```python
from build123d import *

# Parameters (mm, degrees)
F0_W     = 25.4
F0_H     = 28.575
F1_DEPTH = 63.5


with BuildPart() as f1:
    # F0 (on Front) → F1 (new body, symmetric)
    with BuildSketch(Plane.XZ):
        with BuildLine():
            add(Edge.make_bspline(
                [(-41.275, 9.525), (-41.089289, 37.270412), (16.726991, 64.451575), (53.630861, 61.9252)],
                knots=[0, 0, 0, 0, 108.410809, 108.410809, 108.410809, 108.410809], degree=3))
            Line((-41.275, 9.525), (22.225, 9.525))
            Line((22.225, 9.525), (22.225, 30.519339))
            ThreePointArc((22.225, 30.519339), (31.423564, 52.726636), (53.630861, 61.9252))
        make_face()
        Polygon((22.225, 9.525), (-41.275, 9.525), (-41.275, -9.525), (41.275, -9.525), (41.275, 9.525), align=None)
        with BuildLine():
            Line((22.225, 30.519339), (22.225, 9.525))
            Line((22.225, 9.525), (41.275, 9.525))
            Line((41.275, 9.525), (41.275, 30.519339))
            ThreePointArc((41.275, 30.519339), (44.893948, 39.256252), (53.630861, 42.8752))
            Line((53.630861, 42.8752), (60.325, 42.8752))
            Line((60.325, 42.8752), (60.325, 61.9252))
            Line((60.325, 61.9252), (53.630861, 61.9252))
            ThreePointArc((53.630861, 61.9252), (31.423564, 52.726636), (22.225, 30.519339))
        make_face()
        Polygon((60.325, 66.675), (60.325, 61.9252), (60.325, 42.8752), (60.325, 38.1), (85.725, 38.1), (85.725, 66.675), align=None)
        with Locations((98.425, 52.3875)):
            Rectangle(F0_W, F0_H)
    extrude(amount=F1_DEPTH, both=True)


solid = f1.part
```
Work out the finished part from the listing and answer in its coordinate system (mm). A direction names the side the tool comes from. Coordinates: 2 decimals unless noted, no trailing zeros. Order: outer loops, then holes, each group sorted by start corner. A loop starts at its lowest first (then second) coordinate and runs counter-clockwise, first axis right, second up. Notation, with made-up numbers: M -15.75,-10 L 13.25,-10 A26 ccw 13.25,18 Z; hole C -17.75,58.25 d3. An arc over 180 degrees is marked long. Use CSV: the item, a comma, the result in double quotes.
1) Flat-ended cylindrical pins translate along their axes: pin 1 Ø5 at (x, y) = (5.5, -50.5) entering from +Z; pin 2 Ø5 at (y, z) = (-33, 43) entering from -X; pin 3 Ø5 at (y, z) = (-18, 65) entering from -X (3 decimals). Find the tip coordinate at first contact, or state that the pin passes through.
Worked out:
pin 1,"stops at z = 53.98"
pin 2,"stops at x = -18.69"
pin 3,"stops at x = 60.325"
2) Determine the mould class of faces 4 (the face through (-41.275, -1, 0)), 5 (the face through (86, -1, 66.675)), 6 (the face through (57, -1, 42.875)), 7 (the face through (57, -1, 61.925)) for opening direction X: released by +X, released by -X, zero draft, split by the parting line, or undercut.
Worked out:
face 4,"released by -X"
face 5,"zero draft"
face 6,"undercut"
face 7,"undercut"
3) Consider line 1 (X direction, y = 47, z = 3.5) (3 decimals); line 2 (Z direction, x = 53, y = 30.5); line 3 (X direction, y = 49.5, z = 39.5) (3 decimals). Determine where each line is inside the solid, lowest interval first. Write a range as [from, to].
Worked out:
line 1,"x = [-41.275, 41.275]"
line 2,"z = [42.86, 61.97]"
line 3,"x = [-20.14, 45.145], [60.325, 111.125]"
4) Section A-A on z = 3 is taken. Write down the section's boundary in (x, y) (3 decimals).
Worked out:
outline,"M -41.275,-63.5 L 41.275,-63.5 L 41.275,63.5 L -41.275,63.5 Z"
5) For faces 1 (the face through (44.8, -0.89, 39.16)), 2 (the face through (41.275, -1, 10)), 3 (the face through (19, -63.5, 29)), determine the directions among +Z, -Z, +X, -X, +Y, -Y from which every point of the face is accessible in a straight line to the end or side of a thin tool.
Worked out:
face 1,"-Z, +Y, -Y"
face 2,"-Z, +X, +Y, -Y"
face 3,"+Z, -Z, +X, -X, -Y"
